from build123d import *

# Parameters (mm, degrees)
F0_W     = 178.8574159145
F0_H     = 81.6361643374
F1_DEPTH = 254
F2_W     = 23.7848889083
F2_H     = 10.5402404442
F2_W_2   = 26.5901517123
F2_H_2   = 27.3088035174
F2_W_3   = 17.2476675361
F2_H_3   = 17.4872139469
F3_DEPTH = 279.4


with BuildPart() as f1:
    # F0 (on Front) → F1 (new body)
    with BuildSketch(Plane.XZ):
        with Locations((39.3337905407, -5.5660996586)):
            Rectangle(F0_W, F0_H)
    extrude(amount=F1_DEPTH)

    # F2 (on Front) → F3 (join)
    with BuildSketch(Plane.XZ):
        Polygon((-23.7848889083, 18.684970215), (-36.00198403, 18.684970215), (-36.00198403, -33.5371270776), (-23.7848889083, -33.5371270776), (-23.7848889083, -10.5402404442), (-23.7848889083, 0), align=None)
        with Locations((-11.8924444541, -5.2701202221)):
            Rectangle(F2_W, F2_H)
        Polygon((0, 18.4454191476), (0, 0), (0, -10.5402404442), (0, -33.5371270776), (11.1895417795, -33.5371270776), (11.1895417795, 18.4454191476), align=None)
        with Locations((31.1920428649, -19.8827253189)):
            Rectangle(F2_W_2, F2_H_2)
        with Locations((31.3118183985, -19.2838474177)):
            Rectangle(F2_W_3, F2_H_3, mode=Mode.SUBTRACT)
        Polygon((58.2506749504, -4.0445046551), (52.6318475604, -8.144730702), (65.5675977468, -25.8714966476), (55.4336216789, -38.7093556306), (61.0161311924, -42.6400601864), (85.3046610062, -8.144730702), (80.1802054048, -4.0445046551), (68.7108764795, -18.3788526116), align=None)
        Polygon((100.8825037981, 1.7623157246), (94.7928056121, 3.8328145165), (90.7204374671, -8.144730702), (97.5141057214, -8.144730702), align=None)
        Polygon((97.7708830958, -15.8204832481), (89.2352089286, -21.2462227792), (89.2352089286, -33.206935972), (98.6418065629, -39.7368925247), (108.4621548653, -33.206935972), (115.5638098717, -22.9767896235), (108.4621548653, -18.0468988759), (108.4621548653, -22.9767896235), (101.3604998589, -33.206935972), (90.7935802111, -25.8714966476), align=None)
    extrude(amount=F3_DEPTH)


solid = f1.part
Design review of the part built by this model. Coordinates are the model's own, in mm. A direction names the side the tool comes from. Round coordinates to 2 decimals unless told otherwise and drop trailing zeros. Order: outer loops, then holes, each group sorted by start corner. A loop starts at its lowest first (then second) coordinate and runs counter-clockwise, first axis right, second up.
1) Consider section B-B (z = 27). State the section outline as (x, y) points, plus the area to 3 significant figures.
The answers:
outline: (-50.09, -254) - (128.76, -254) - (128.76, 0) - (-50.09, 0) - close
area: 45,400 mm2
2) Draft analysis for pull direction X (two halves, no side actions). For faces 5 (the flat face through (112.063, -266.522, -20.546)), 6 (the flat face through (59.009, -266.522, -16.884)), 7 (the flat face through (69, -279.4, -19)), state which applies: released by +X, released by -X, zero draft, split by the parting line, or undercut.
The answers:
face 5: released by +X
face 6: undercut
face 7: zero draft
3) For L1, parallel to Z at x = 34, y = -254.5; L2, parallel to X at y = -263.5, z = 4; L3, parallel to Y at x = -31, z = -39.5, list the stretches that pass through material, from the lowest coordinate up.
The answers:
L1: z = -33.54 to -28.03, -10.54 to -6.23
L2: x = -36 to -23.78, 0 to 11.19
L3: y = -254 to 0
4) Machinability: for faces 1 (the flat face through (104.96, -266.52, -28.02)), 2 (the flat face through (58.19, -266.52, -40.65)), 3 (the flat face through (31, -267, -28.027)), 4 (the flat face through (93.873, -266.522, -36.426)), which of the approach directions +Z, -Z, +X, -X, +Y, -Y give a long, thin tool a straight path to every point of the face, cutting with its end or side? Answer none if there is none.
The answers:
face 1: +Z, -Y
face 2: -Z, -X, -Y
face 3: -Y
face 4: -Z, -Y
5) Consider section A-A (x = -9.5). State the section outline as (y, z) points.
The answers:
outline: (-279.4, -10.54) - (-254, -10.54) - (-254, -46.38) - (0, -46.38) - (0, 35.25) - (-254, 35.25) - (-254, 0) - (-279.4, 0) - close
6) Clearance check with flat-ended pins moving along their axes: pin 1 Ø6 at (x, z) = (97, -4.5) entering from +Y; pin 2 Ø1.5 at (y, z) = (-263.5, -20.5) entering from -X; pin 3 Ø12.5 at (x, y) = (7.5, -263.5) entering from -Z; pin 4 Ø14 at (x, y) = (30, -264.5) entering from +Z. State where each tip first meets the part, or that it passes through.
The answers:
pin 1: stops at y = 0
pin 2: stops at x = -36
pin 3: stops at z = -33.54
pin 4: stops at z = -6.23
